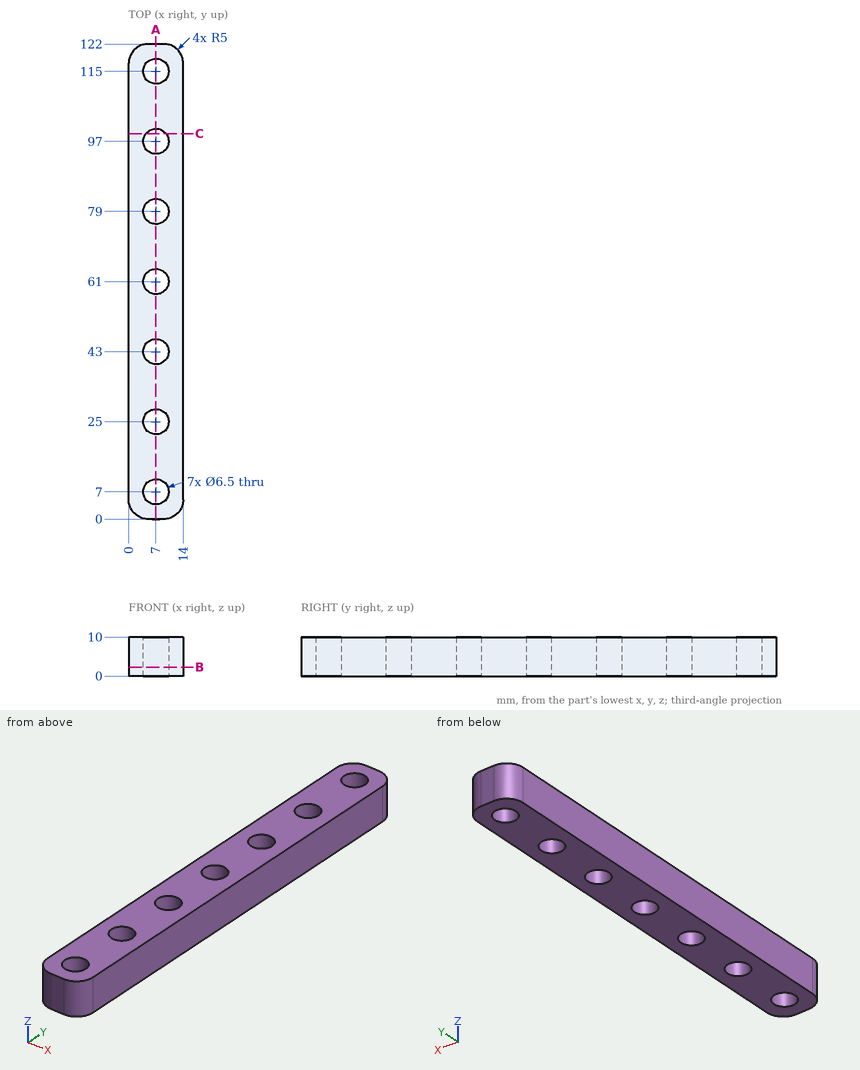
Print and shaded views of the part. All mm, measured from the part's lowest x, y and z. Coordinates: 2 decimals unless noted, no trailing zeros. Write each loop counter-clockwise with the first axis right and the second up, starting at its lowest first coordinate (ties: lowest second). Pieces come first, ordered by that corner, then holes.
(1) Cut at B-B, the plane z = 2.25. List the corners of the cut face in (x, y).
(2) Cut at C-C, the plane y = 99. List the corners of the cut face in (x, z).
(3) Drill centre lines: probe 1 along X at (y, z) = (63, 8.5); probe 2 along Y at (x, z) = (2, 7.25); probe 3 along Y at (x, z) = (3, 3.5). Where is each one in solid material? Low to high.
(4) Cut at A-A, the plane x = 7. Count the separate pieces of the cut face and the enclosed holes in it, and give its area (3 significant figures).
(5) Flat gauge pin, fed straight in: pin 1 (4 mm diameter, centred on x = 7, y = 25, fed in from +Z). Where does the tip first touch, or does it go through?
Geometry says:
1. outline: (0, 5) arc R5 ccw to (5, 0) - (9, 0) arc R5 ccw to (14, 5) - (14, 117) arc R5 ccw to (9, 122) - (5, 122) arc R5 ccw to (0, 117) - close; hole circle Ø6.5 at (7, 7); hole circle Ø6.5 at (7, 25); hole circle Ø6.5 at (7, 43); hole circle Ø6.5 at (7, 61); hole circle Ø6.5 at (7, 79); hole circle Ø6.5 at (7, 97); hole circle Ø6.5 at (7, 115)
2. outline: (0, 0) - (4.44, 0) - (4.44, 10) - (0, 10) - close; (9.56, 0) - (14, 0) - (14, 10) - (9.56, 10) - close
3. probe 1: x = 0 to 4.44, 9.56 to 14
3. probe 2: y = 1 to 121
3. probe 3: y = 0.42 to 121.58
4. separate pieces: 8
4. enclosed holes: 0
4. area: 765 mm2
5. pin 1: passes through
